```python
from build123d import *

# Parameters (mm, degrees)
BOSS_EXTRUDE1_DEPTH      = 9
BOSS_EXTRUDE1_DEPTH_BACK = 9
SKETCH1_W                = 53
SKETCH1_H                = 17
SKETCH2_W                = 45
SKETCH2_H                = 18
BOSS_EXTRUDE2_DEPTH      = 3
SKETCH3_W                = 8
SKETCH3_H                = 10
BOSS_EXTRUDE3_DEPTH      = 9
SKETCH4_W                = 12
SKETCH4_H                = 12
BOSS_EXTRUDE4_DEPTH      = 146
CUT_EXTRUDE1_REACH       = 149.028
SKETCH6_R                = 2.125
FILLET2_R                = 2
FILLET3_R                = 1
SKETCH7_R                = 4.5
CUT_EXTRUDE2_DEPTH       = 140
FILLET4_R                = 1


with BuildPart() as part:
    # Sketch1 → Boss-Extrude1 (new, two sides: drawn at the far end of the back side and taken through both)
    with BuildSketch(Plane.XY.offset(-BOSS_EXTRUDE1_DEPTH_BACK)):
        with Locations((26.5, 0)):
            Rectangle(SKETCH1_W, SKETCH1_H)
    extrude(amount=BOSS_EXTRUDE1_DEPTH + BOSS_EXTRUDE1_DEPTH_BACK)

    # Sketch2 → Boss-Extrude2 (add)
    with BuildSketch(Plane(origin=(0, 8.5, 0), x_dir=(1, 0, 0), z_dir=(0, 1, 0))):
        with Locations((30.5, 0)):
            Rectangle(SKETCH2_W, SKETCH2_H)
    extrude(amount=BOSS_EXTRUDE2_DEPTH)

    # Sketch3 → Boss-Extrude3 (add)
    with BuildSketch(Plane(origin=(53, 0, 0), x_dir=(0, 0, -1), z_dir=(1, 0, 0))):
        Rectangle(SKETCH3_W, SKETCH3_H)
    extrude(amount=BOSS_EXTRUDE3_DEPTH)

    # Sketch4 → Boss-Extrude4 (add)
    with BuildSketch(Plane.ZY):
        Rectangle(SKETCH4_W, SKETCH4_H)
    extrude(amount=BOSS_EXTRUDE4_DEPTH)

    # Sketch6 → Cut-Extrude1 (cut, up to next)
    with BuildSketch(Plane.XY.offset(4), mode=Mode.PRIVATE) as cut_extrude1_sk1:
        with Locations((57.5, 0)):
            Circle(SKETCH6_R)
    cut_extrude1_tool1 = extrude(cut_extrude1_sk1.sketch, amount=-CUT_EXTRUDE1_REACH, mode=Mode.PRIVATE) & part.part
    add(cut_extrude1_tool1.solids().sort_by_distance((57.5, 0, 4))[0], mode=Mode.SUBTRACT)

    # Fillet2
    fillet2_edges = [part.edges().sort_by_distance(p)[0] for p in [
        (26.5, -8.5, -9),
    ]]
    fillet(fillet2_edges, radius=FILLET2_R)
    fillet2_2_edges = [part.edges().sort_by_distance(p)[0] for p in [
        (26.5, -8.5, 9),
    ]]
    fillet(fillet2_2_edges, radius=FILLET2_R)
    fillet2_3_edges = [part.edges().sort_by_distance(p)[0] for p in [
        (30.5, 11.5, -9),
    ]]
    fillet(fillet2_3_edges, radius=FILLET2_R)
    fillet2_4_edges = [part.edges().sort_by_distance(p)[0] for p in [
        (30.5, 11.5, 9),
    ]]
    fillet(fillet2_4_edges, radius=FILLET2_R)
    fillet2_5_edges = [part.edges().sort_by_distance(p)[0] for p in [
        (53, 1.5, -9),
    ]]
    fillet(fillet2_5_edges, radius=FILLET2_R)
    fillet2_6_edges = [part.edges().sort_by_distance(p)[0] for p in [
        (0, 8.5, 0),
    ]]
    fillet(fillet2_6_edges, radius=FILLET2_R)
    fillet2_7_edges = [part.edges().sort_by_distance(p)[0] for p in [
        (0, -8.5, 0),
    ]]
    fillet(fillet2_7_edges, radius=FILLET2_R)
    fillet2_8_edges = [part.edges().sort_by_distance(p)[0] for p in [
        (8, 11.5, 0),
    ]]
    fillet(fillet2_8_edges, radius=FILLET2_R)
    fillet2_9_edges = [part.edges().sort_by_distance(p)[0] for p in [
        (62, 0, -4),
    ]]
    fillet(fillet2_9_edges, radius=FILLET2_R)
    fillet2_10_edges = [part.edges().sort_by_distance(p)[0] for p in [
        (62, 0, 4),
    ]]
    fillet(fillet2_10_edges, radius=FILLET2_R)
    fillet2_11_edges = [part.edges().sort_by_distance(p)[0] for p in [
        (56.5, -5, 4),
    ]]
    fillet(fillet2_11_edges, radius=FILLET2_R)
    fillet2_12_edges = [part.edges().sort_by_distance(p)[0] for p in [
        (56.5, 5, -4),
    ]]
    fillet(fillet2_12_edges, radius=FILLET2_R)

    # Fillet3
    fillet3_edges = [part.edges().sort_by_distance(p)[0] for p in [
        (53, -5, 0),
        (53, 0, 4),
        (53, 5, 0),
        (53, 0, -4),
        (53, 4.414213562, 3.414213562),
        (53, 4.414213562, -3.414213562),
        (53, -4.414213562, -3.414213562),
        (53, -4.414213562, 3.414213562),
    ]]
    fillet(fillet3_edges, radius=FILLET3_R)

    # Sketch7 → Cut-Extrude2 (cut)
    with BuildSketch(Plane.ZY.offset(146)):
        with Locations(Location((0, 0, 0), (0, 0, 270))):
            Circle(SKETCH7_R)
    extrude(amount=-CUT_EXTRUDE2_DEPTH, mode=Mode.SUBTRACT)

    # Fillet4
    fillet4_edges = [part.edges().sort_by_distance(p)[0] for p in [
        (-73, 6, -6),
        (-73, -6, -6),
        (-73, -6, 6),
        (-73, 6, 6),
        (-146, 0, -6),
        (-146, -6, 0),
        (-146, 0, 6),
        (-146, 6, 0),
    ]]
    fillet(fillet4_edges, radius=FILLET4_R)


solid = part.part
```
Can you work these out from the model? Positions are in its coordinate system, mm. A direction names the side the tool comes from. Round coordinates to 2 decimals unless told otherwise and drop trailing zeros. Order: outer loops, then holes, each group sorted by start corner. A loop starts at its lowest first (then second) coordinate and runs counter-clockwise, first axis right, second up. Notation, with made-up numbers: (-4.5, 56) -> (10.5, 56) arc R11 cw to (10.5, 67) -> close; hole circle Ø1 at (77, 69). An arc over 180 degrees is marked (long way). Return JSON: item names as keys, results as strings. Group by question number.
1. If we section it at D-D, the plane x = -22.5: Write out the boundary of the cut face in (y, z).
2. Which directions (+Z, -Z, +X, -X, +Y, -Y) give clear straight access to the entire face, cutting with the end or side of a thin tool? Please do faces 5 (the face through (57, -5, 0)), 6 (the face through (55.6, -1.4, -4)), 7 (the face through (5, 8.5, 0)), 8 (the face through (-6, 0, 0)), 9 (the face through (57, 5, 0)).
3. We'd pull the mould along X, two halves only. Please class faces 1 (the face through (53, 7, 0)), 2 (the face through (0, -0.5, 6.2)), 3 (the face through (55.377, 0.093, 0.056)), 4 (the face through (26, -8.5, 0)): released by +X, released by -X, zero draft, split by the parting line, or undercut.
4. I need wall thicknesses on line 1 (Y direction, x = 57.5, z = -1.75) (3 decimals); line 2 (Y direction, x = 5, z = 3); line 3 (Z direction, x = -57, y = 3.75). Which ranges of each line are inside material? Lowest first, please. Write a range as [from, to].
5. If we section it at B-B, the plane x = 57.5: Write out the boundary of the cut face in (y, z) (3 decimals).
6. Will these pins go through, and if not, where does the flat tip stop? pin 1 (5 mm diameter, centred on x = -78.5, y = -2, fed in from -Z); pin 2 (2 mm diameter, centred on x = 56.5, z = 1, fed in from +Y); pin 3 (5 mm diameter, centred on x = -81.5, y = 7, fed in from +Z).
Output values:
{
 "1": {"outline": "(-6, -5) arc R1 ccw to (-5, -6) -> (5, -6) arc R1 ccw to (6, -5) -> (6, 5) arc R1 ccw to (5, 6) -> (-5, 6) arc R1 ccw to (-6, 5) -> close; hole circle Ø9 at (0, 0)"},
 "2": {"face 5": "+Z, -Z, +X, -Y", "face 6": "-Z, +X, +Y, -Y", "face 7": "+Z, -Z, -X, +Y", "face 8": "-X", "face 9": "+Z, -Z, +X, +Y"},
 "3": {"face 1": "released by +X", "face 2": "released by -X", "face 3": "undercut", "face 4": "zero draft"},
 "4": {"line 1": "[-5, -2.125], [2.125, 5]", "line 2": "[-8.5, 8.5]", "line 3": "[-6, -2.49], [2.49, 6]"},
 "5": {"outline": "(-5, -2) arc R2 ccw to (-3, -4) -> (-2.125, -4) -> (-2.125, 4) -> (-3, 4) arc R2 ccw to (-5, 2) -> close; (2.125, -4) -> (3, -4) arc R2 ccw to (5, -2) -> (5, 2) arc R2 ccw to (3, 4) -> (2.125, 4) -> close"},
 "6": {"pin 1": "z = -6", "pin 2": "y = 5", "pin 3": "z = 6"}
}
